```python
from build123d import *

# Parameters (mm, degrees)
SKETCH2_W           = 50.8
SKETCH2_H           = 25.4
SKETCH2_W_2         = 45.72
SKETCH2_H_2         = 20.32
BOSS_EXTRUDE1_DEPTH = 635
SKETCH3_R           = 2.032
CUT_EXTRUDE1_DEPTH  = 638.155342126
SKETCH4_R           = 2.032
CUT_EXTRUDE2_DEPTH  = 637.015188498
SKETCH5_R           = 14.351
SKETCH5_R_2         = 2.479261189
CUT_EXTRUDE3_DEPTH  = 637.015188498
SKETCH6_W           = 50.8
SKETCH6_H           = 25.4
CUT_EXTRUDE4_DEPTH  = 355.6
SKETCH12_W          = 50.8
SKETCH12_H          = 25.4
CUT_EXTRUDE9_DEPTH  = 38.1


with BuildPart() as part:
    # Sketch2 → Boss-Extrude1 (new body)
    with BuildSketch(Plane(origin=(0, 0, 0), x_dir=(1, 0, 0), z_dir=(0, 1, 0))):
        Rectangle(SKETCH2_W, SKETCH2_H)
        Rectangle(SKETCH2_W_2, SKETCH2_H_2, mode=Mode.SUBTRACT)
    extrude(amount=BOSS_EXTRUDE1_DEPTH)

    # Sketch3 → Cut-Extrude1 (cut, through all)
    with BuildSketch(Plane(origin=(25.4, 0, 0), x_dir=(0, 0, -1), z_dir=(1, 0, 0))):
        Circle(SKETCH3_R)
        with Locations((0, 12.7)):
            Circle(SKETCH3_R)
        with Locations((0, 25.4)):
            Circle(SKETCH3_R)
        with Locations((0, 38.1)):
            Circle(SKETCH3_R)
        with Locations((0, 50.8)):
            Circle(SKETCH3_R)
        with Locations((0, 63.5)):
            Circle(SKETCH3_R)
        with Locations((0, 76.2)):
            Circle(SKETCH3_R)
        with Locations((0, 88.9)):
            Circle(SKETCH3_R)
        with Locations((0, 101.6)):
            Circle(SKETCH3_R)
        with Locations((0, 114.3)):
            Circle(SKETCH3_R)
        with Locations((0, 127)):
            Circle(SKETCH3_R)
        with Locations((0, 139.7)):
            Circle(SKETCH3_R)
        with Locations((0, 152.4)):
            Circle(SKETCH3_R)
        with Locations((0, 165.1)):
            Circle(SKETCH3_R)
        with Locations((0, 177.8)):
            Circle(SKETCH3_R)
        with Locations((0, 190.5)):
            Circle(SKETCH3_R)
        with Locations((0, 203.2)):
            Circle(SKETCH3_R)
        with Locations((0, 215.9)):
            Circle(SKETCH3_R)
        with Locations((0, 228.6)):
            Circle(SKETCH3_R)
        with Locations((0, 241.3)):
            Circle(SKETCH3_R)
        with Locations((0, 254)):
            Circle(SKETCH3_R)
        with Locations((0, 266.7)):
            Circle(SKETCH3_R)
        with Locations((0, 279.4)):
            Circle(SKETCH3_R)
        with Locations((0, 292.1)):
            Circle(SKETCH3_R)
        with Locations((0, 304.8)):
            Circle(SKETCH3_R)
        with Locations((0, 317.5)):
            Circle(SKETCH3_R)
        with Locations((0, 330.2)):
            Circle(SKETCH3_R)
        with Locations((0, 342.9)):
            Circle(SKETCH3_R)
        with Locations((0, 355.6)):
            Circle(SKETCH3_R)
        with Locations((0, 368.3)):
            Circle(SKETCH3_R)
        with Locations((0, 381)):
            Circle(SKETCH3_R)
        with Locations((0, 393.7)):
            Circle(SKETCH3_R)
        with Locations((0, 406.4)):
            Circle(SKETCH3_R)
        with Locations((0, 419.1)):
            Circle(SKETCH3_R)
        with Locations((0, 431.8)):
            Circle(SKETCH3_R)
        with Locations((0, 444.5)):
            Circle(SKETCH3_R)
        with Locations((0, 457.2)):
            Circle(SKETCH3_R)
        with Locations((0, 469.9)):
            Circle(SKETCH3_R)
        with Locations((0, 482.6)):
            Circle(SKETCH3_R)
        with Locations((0, 495.3)):
            Circle(SKETCH3_R)
        with Locations((0, 508)):
            Circle(SKETCH3_R)
        with Locations((0, 520.7)):
            Circle(SKETCH3_R)
        with Locations((0, 533.4)):
            Circle(SKETCH3_R)
        with Locations((0, 546.1)):
            Circle(SKETCH3_R)
        with Locations((0, 558.8)):
            Circle(SKETCH3_R)
        with Locations((0, 571.5)):
            Circle(SKETCH3_R)
        with Locations((0, 584.2)):
            Circle(SKETCH3_R)
        with Locations((0, 596.9)):
            Circle(SKETCH3_R)
        with Locations((0, 609.6)):
            Circle(SKETCH3_R)
        with Locations((0, 622.3)):
            Circle(SKETCH3_R)
    extrude(amount=-CUT_EXTRUDE1_DEPTH, mode=Mode.SUBTRACT)

    # Sketch4 → Cut-Extrude2 (cut, through all)
    with BuildSketch(Plane.XY.offset(12.7)):
        with Locations((-12.7, 12.7)):
            Circle(SKETCH4_R)
        with Locations((0, 12.7)):
            Circle(SKETCH4_R)
        with Locations((12.7, 12.7)):
            Circle(SKETCH4_R)
    extrude(amount=-CUT_EXTRUDE2_DEPTH, mode=Mode.SUBTRACT)

    # Sketch5 → Cut-Extrude3 (cut, through all)
    with BuildSketch(Plane.XY.offset(12.7)):
        with Locations((0, 87.63)):
            Circle(SKETCH5_R)
        with Locations((-19.05, 106.68)):
            Circle(SKETCH5_R_2)
        with Locations((19.05, 106.68)):
            Circle(SKETCH5_R_2)
        with Locations((19.05, 68.58)):
            Circle(SKETCH5_R_2)
        with Locations((-19.05, 68.58)):
            Circle(SKETCH5_R_2)
    extrude(amount=-CUT_EXTRUDE3_DEPTH, mode=Mode.SUBTRACT)

    # Sketch6 → Cut-Extrude4 (cut)
    with BuildSketch(Plane(origin=(0, 635, 0), x_dir=(1, 0, 0), z_dir=(0, 1, 0))):
        Rectangle(SKETCH6_W, SKETCH6_H)
    extrude(amount=-CUT_EXTRUDE4_DEPTH, mode=Mode.SUBTRACT)

    # Sketch12 → Cut-Extrude9 (cut)
    with BuildSketch(Plane(origin=(0, 279.4, 0), x_dir=(1, 0, 0), z_dir=(0, 1, 0))):
        Rectangle(SKETCH12_W, SKETCH12_H)
    extrude(amount=-CUT_EXTRUDE9_DEPTH, mode=Mode.SUBTRACT)


solid = part.part
```
Here's how the part is built. I have some questions about the finished solid (model axes, mm). Coordinates: 2 decimals unless noted, no trailing zeros. Order: outer loops, then holes, each group sorted by start corner. A loop starts at its lowest first (then second) coordinate and runs counter-clockwise, first axis right, second up. Notation, with made-up numbers: (-30, 44) - (27, 44) arc R10 ccw to (27, 53) - close; hole circle Ø3 at (9, 50.25). An arc over 180 degrees is marked (long way). One line per question, with ' | ' between items.
(1) If I drill on L1, parallel to Y at x = 0, z = 11.25; L2, parallel to X at y = 98.5, z = 3.5; L3, parallel to Z at x = 16, y = 112, over which ranges is the centre line in solid material (lowest first)?
Report:
L1: y = 0 to 10.67, 14.73 to 73.28, 101.98 to 241.3 | L2: x = -25.4 to -22.86, 22.86 to 25.4 | L3: z = -12.7 to -10.16, 10.16 to 12.7
(2) Suppose I cut it at D-D on x = -19.05. List the corners of the cut face in (y, z) for me, and give its area (3 significant figures).
Report:
outline: (0, -12.7) - (66.1, -12.7) - (66.1, -10.16) - (0, -10.16) - close; (0, 10.16) - (66.1, 10.16) - (66.1, 12.7) - (0, 12.7) - close; (71.06, -12.7) - (104.2, -12.7) - (104.2, -10.16) - (71.06, -10.16) - close; (71.06, 10.16) - (104.2, 10.16) - (104.2, 12.7) - (71.06, 12.7) - close; (109.16, -12.7) - (241.3, -12.7) - (241.3, -10.16) - (109.16, -10.16) - close; (109.16, 10.16) - (241.3, 10.16) - (241.3, 12.7) - (109.16, 12.7) - close | area: 1,180 mm2
(3) Suppose I cut it at B-B on z = -8. List the corners of the cut face in (x, y) for me, and give its area (3 significant figures).
Report:
outline: (-25.4, 0) - (-22.86, 0) - (-22.86, 241.3) - (-25.4, 241.3) - close; (22.86, 0) - (25.4, 0) - (25.4, 241.3) - (22.86, 241.3) - close | area: 1,230 mm2
(4) If we mould it in two halves opening along Y, with no side actions, what happens to faces 1 (the flat face through (0, 0, 11)), 2 (the flat face through (25.4, 119, 0)), 3 (the cylindrical face through (-24.112, 10.716, 0.44)), 4 (the cylindrical face through (24.148, 217.915, 0.265))? For each: pulls with the +Y half, pulls with the -Y half, needs draft (parallel to the pull), parting line crosses it, or undercut.
Report:
face 1: pulls with the -Y half | face 2: needs draft | face 3: undercut | face 4: undercut
(5) Suppose I cut it at C-C on y = 190.5. List the corners of the cut face in (x, z) for me, and give its area (3 significant figures).
Report:
outline: (-25.4, -12.7) - (25.4, -12.7) - (25.4, -2.03) - (22.86, -2.03) - (22.86, -10.16) - (-22.86, -10.16) - (-22.86, -2.03) - (-25.4, -2.03) - close; (-25.4, 2.03) - (-22.86, 2.03) - (-22.86, 10.16) - (22.86, 10.16) - (22.86, 2.03) - (25.4, 2.03) - (25.4, 12.7) - (-25.4, 12.7) - close | area: 341 mm2
(6) Suppose I cut it at A-A on x = 0. List the corners of the cut face in (y, z) for me.
Report:
outline: (0, -12.7) - (10.67, -12.7) - (10.67, -10.16) - (0, -10.16) - close; (0, 10.16) - (10.67, 10.16) - (10.67, 12.7) - (0, 12.7) - close; (14.73, -12.7) - (73.28, -12.7) - (73.28, -10.16) - (14.73, -10.16) - close; (14.73, 10.16) - (73.28, 10.16) - (73.28, 12.7) - (14.73, 12.7) - close; (101.98, -12.7) - (241.3, -12.7) - (241.3, -10.16) - (101.98, -10.16) - close; (101.98, 10.16) - (241.3, 10.16) - (241.3, 12.7) - (101.98, 12.7) - close
